```python
from build123d import *

# Parameters (mm, degrees)
SKETCH_1_W          = 68
SKETCH_1_H          = 58
SKETCH_1_R          = 1.25
EXTRUDE_1_DEPTH     = 2
SKETCH_2_W          = 2
SKETCH_2_H          = 40
EXTRUDE_2_DEPTH     = 68
SKETCH_3_W          = 9
SKETCH_3_H          = 50
CUT_EXTRUDE_1_DEPTH = 10
FILLET_1_R          = 3


with BuildPart() as part:
    # 草图1 → 凸台-拉伸1 (new body)
    with BuildSketch(Plane.XY):
        with Locations((34, 29)):
            Rectangle(SKETCH_1_W, SKETCH_1_H)
        with Locations((48, 27)):
            Circle(SKETCH_1_R, mode=Mode.SUBTRACT)
        with Locations(Location((20, 27, 0), (0, 0, 180))):
            Circle(SKETCH_1_R, mode=Mode.SUBTRACT)
        with Locations((48, 47)):
            Circle(SKETCH_1_R, mode=Mode.SUBTRACT)
        with Locations(Location((20, 47, 0), (0, 0, 180))):
            Circle(SKETCH_1_R, mode=Mode.SUBTRACT)
    extrude(amount=EXTRUDE_1_DEPTH)

    # 草图2 → 凸台-拉伸2 (add)
    with BuildSketch(Plane(origin=(68, 0, 0), x_dir=(0, 0, -1), z_dir=(1, 0, 0))):
        with Locations((-1, -20)):
            Rectangle(SKETCH_2_W, SKETCH_2_H)
    extrude(amount=-EXTRUDE_2_DEPTH)

    # 草图3 → 切除-拉伸1 (cut)
    with BuildSketch(Plane.XY.offset(2)):
        with Locations((4.5, -15)):
            Rectangle(SKETCH_3_W, SKETCH_3_H)
        with Locations((63.5, -15)):
            Rectangle(SKETCH_3_W, SKETCH_3_H)
    extrude(amount=-CUT_EXTRUDE_1_DEPTH, mode=Mode.SUBTRACT)

    # 圆角1
    fillet_1_edges = [part.edges().sort_by_distance(p)[0] for p in [
        (59, -40, 1),
        (9, -40, 1),
        (0, 10, 1),
        (9, 10, 1),
        (68, 10, 1),
        (59, 10, 1),
        (0, 58, 1),
        (68, 58, 1),
    ]]
    fillet(fillet_1_edges, radius=FILLET_1_R)


solid = part.part
```
The model under review builds one solid part; all positions refer to its coordinate system, in mm. A direction names the side the tool comes from. Give positions to 0.01 mm unless a question says otherwise; leave off trailing zeros. Loops run counter-clockwise (first coordinate to the right, second up) from the corner with the lowest first, then second, coordinate; pieces in that order, holes last. Notation, with made-up numbers: (-6.75, 64.5) - (4.25, 64.5) arc R25 ccw to (4.25, 98.5) - close; hole circle Ø3 at (44, -11.5). An arc over 180 degrees is marked (long way). Answer as a JSON object with one key per item and string values.
Q1. Add section A-A on y = 27. State the section outline as (x, z) points, plus the area to 3 significant figures.
Worked out:
{"outline": "(0, 0) - (18.75, 0) - (18.75, 2) - (0, 2) - close; (21.25, 0) - (46.75, 0) - (46.75, 2) - (21.25, 2) - close; (49.25, 0) - (68, 0) - (68, 2) - (49.25, 2) - close", "area": "126 mm^2"}
Q2. Add section D-D on y = -19.5. State the section outline as (x, z) points.
Worked out:
{"outline": "(9, 0) - (59, 0) - (59, 2) - (9, 2) - close"}
Q3. For faces 1 (the flat face through (4, 10, 1)), 2 (the flat face through (63, 10, 1)), 3 (the cylindrical face through (67.14, 57.1, 1.01)), list the 3-axis set-ups (+Z, -Z, +X, -X, +Y, -Y) from which the entire face can be reached by the end or side of a thin tool; tool diameter is ignored.
Worked out:
{"face 1": "+Z, -Z, -X, -Y", "face 2": "+Z, -Z, +X, -Y", "face 3": "+Z, -Z, +X, +Y"}
Q4. Add section C-C on z = 1. State the section outline as (x, y) points.
Worked out:
{"outline": "(0, 13) arc R3 ccw to (3, 10) - (6, 10) arc R3 cw to (9, 7) - (9, -37) arc R3 ccw to (12, -40) - (56, -40) arc R3 ccw to (59, -37) - (59, 7) arc R3 cw to (62, 10) - (65, 10) arc R3 ccw to (68, 13) - (68, 55) arc R3 ccw to (65, 58) - (3, 58) arc R3 ccw to (0, 55) - close; hole circle Ø2.5 at (20, 27); hole circle Ø2.5 at (20, 47); hole circle Ø2.5 at (48, 27); hole circle Ø2.5 at (48, 47)"}
Q5. Add section B-B on x = 20. State the section outline as (y, z) points.
Worked out:
{"outline": "(-40, 0) - (25.75, 0) - (25.75, 2) - (-40, 2) - close; (28.25, 0) - (45.75, 0) - (45.75, 2) - (28.25, 2) - close; (48.25, 0) - (58, 0) - (58, 2) - (48.25, 2) - close"}
Q6. Insertion check: pin 1 (1 mm diameter, centred on x = 4, z = 0.5, fed in from -Y); pin 2 (3 mm diameter, centred on x = 20, y = 47, fed in from +Z); pin 3 (1 mm diameter, centred on y = -20, z = 1, fed in from +X). Each pin has a flat end and moves straight along its axis. Give the tip position at first contact, or say it passes through.
Worked out:
{"pin 1": "stops at y = 10", "pin 2": "stops at z = 2", "pin 3": "stops at x = 59"}
Q7. To check wall thickness, follow line 1 along Y through (x, z) = (20, 1); line 2 along Y through (x, z) = (47, 1.4); line 3 along X through (y, z) = (26, 0.6). State the ranges of each line that lie inside material, in increasing order.
Worked out:
{"line 1": "y = -40 to 25.75, 28.25 to 45.75, 48.25 to 58", "line 2": "y = -40 to 26.25, 27.75 to 46.25, 47.75 to 58", "line 3": "x = 0 to 19.25, 20.75 to 47.25, 48.75 to 68"}
Q8. Mouldability with a two-part tool opening along Y and no side actions: class faces 4 (the cylindrical face through (18.845, 27.479, 0.986)), 5 (the cylindrical face through (0.86, 10.9, 0.99)), 6 (the flat face through (34, 58, 1)), 7 (the flat face through (0, 34, 1)) as +Y half, -Y half, draft (parallel to the pull), parting line (faces both ways), or undercut.
Worked out:
{"face 4": "undercut", "face 5": "-Y half", "face 6": "+Y half", "face 7": "draft"}
